Verification items for the finished model (mm, model axes). A direction names the side the tool comes from. Round coordinates to 2 decimals unless told otherwise and drop trailing zeros. Return JSON: item names as keys, results as strings. Group by question number.
Item 1: Draft check along Z on faces 1 (the cylindrical face through (42.14, 62.5, -36.07)), 2 (the flat face through (37.24, 65.621, -31.428)), 3 (the flat face through (38.784, 62, -36)), 4 (the cylindrical face through (34.085, 61.746, -36.101)). Enter one of: pulls with the +Z half, pulls with the -Z half, needs draft (parallel to the pull), parting line crosses it, or undercut.
Item 2: Scan lines: probe 1 along Y at (x, z) = (38.25, -31.25); probe 2 along Y at (x, z) = (38, -37.75); probe 3 along X at (y, z) = (63.75, -31.75). Record each from-to range of solid material in increasing order. Write a range as from..to.
Item 3: Access from +Z, -Z, +X, -X, +Y, -Y to the whole of each face (thin tool, end or side, straight path). Record for faces 5 (the flat face through (36.467, 64.968, -32.186)), 6 (the flat face through (39.018, 58.55, -39.854)).
Item 4: Depth check by flat-ended pin: pin 1 Ø4 at (y, z) = (64.5, -33.5) entering from +X; pin 2 Ø1 at (y, z) = (60.5, -36) entering from -X; pin 3 Ø1 at (x, z) = (34, -35.5) entering from +Y. Enter the tip coordinate at first touch or a pass-through.
```python
from build123d import *

# Parameters (mm, degrees)
SKETCH2_R           = 5
BOSS_EXTRUDE1_DEPTH = 10
SKETCH3_R           = 5
BOSS_EXTRUDE2_DEPTH = 1
CHAMFER1_SIZE       = 1


with BuildPart() as part:
    # Sketch2 → Boss-Extrude1 (new body)
    with BuildSketch(Plane(origin=(0, 4.567005967, 5.442745768), x_dir=(1, 0, 0), z_dir=(0, 0.6427876096865435, 0.7660444431189747))):
        with Locations(Location((37.184001138, 70.413914347, 0), (0, 0, 270))):
            Circle(SKETCH2_R)
        with BuildLine():
            Line((38.784001138, 67.758730476), (38.784001138, 73.069098218))
            ThreePointArc((38.784001138, 73.069098218), (34.084000914, 70.413914347), (38.784001138, 67.758730476))
        make_face(mode=Mode.SUBTRACT)
    extrude(amount=BOSS_EXTRUDE1_DEPTH)

    # Sketch3 → Boss-Extrude2 (add)
    with BuildSketch(Plane(origin=(0, 10.994882064, 13.1031902), x_dir=(1, 0, 0), z_dir=(0, 0.6427876096865434, 0.7660444431189747))):
        with Locations(Location((37.184001138, 70.413914347, 0), (0, 0, 270))):
            Circle(SKETCH3_R)
    extrude(amount=BOSS_EXTRUDE2_DEPTH)

    # Chamfer1
    chamfer1_edges = [part.edges().sort_by_distance(p)[0] for p in [
        (37.184001138, 69.408079693, -34.605895097),
        (37.184001138, 62.337415986, -43.032383972),
    ]]
    chamfer(chamfer1_edges, length=CHAMFER1_SIZE)


solid = part.part
```
Recorded:
{
 "1": {"face 1": "parting line crosses it", "face 2": "pulls with the +Z half", "face 3": "undercut", "face 4": "undercut"},
 "2": {"probe 1": "59.32..61.9, 63.85..65.41", "probe 2": "56.04..56.34, 64.15..66.68", "probe 3": "32.32..34.31, 38.78..42.05"},
 "3": {"face 5": "none", "face 6": "-Z, +X, -X, -Y"},
 "4": {"pin 1": "x = 42.18", "pin 2": "x = 32.2", "pin 3": "y = 67.81"}
}
